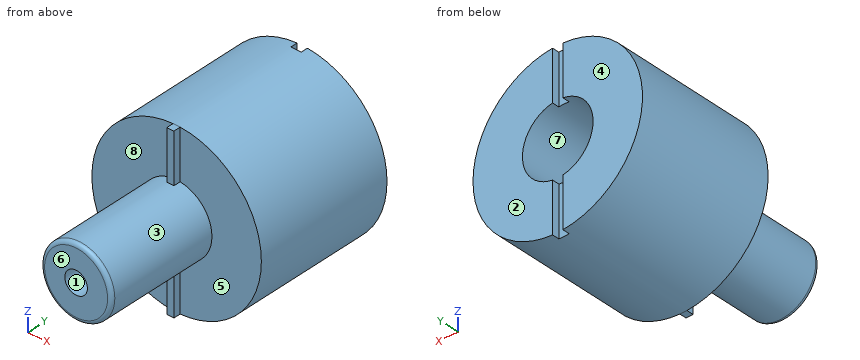
from build123d import *

# Parameters (mm, degrees)
F0_R      = 19.05
F1_DEPTH  = 31.75
F2_R      = 7.9375
F3_DEPTH  = 25.4
F4_R      = 0.8584943428
F6_DEPTH  = 1.5875
F8_DEPTH  = 1.5875
F11_R     = 7.9375
F12_DEPTH = 25.4
F9_R      = 2.54
F13_DEPTH = 31.75
F14_DEPTH = 1.5875


with BuildPart() as f1:
    # F0 (on Front) → F1 (new body)
    with BuildSketch(Plane.XZ):
        Circle(F0_R)
    extrude(amount=F1_DEPTH)

    # F2 (on face) → F3 (join)
    with BuildSketch(Plane.XZ.offset(31.75)):
        Circle(F2_R)
    extrude(amount=F3_DEPTH)

    # F4
    f4_edges = [f1.edges().sort_by_distance(p)[0] for p in [
        (-7.9375, -57.15, 0),
    ]]
    fillet(f4_edges, radius=F4_R)

    # F5 (on face) → F6 (join)
    with BuildSketch(Plane.XZ.offset(31.75)):
        with BuildLine():
            Line((0.79375, 19.0334563581), (-0.79375, 19.0334563581))
            Line((-0.79375, 19.0334563581), (-0.79375, 7.897712782))
            ThreePointArc((-0.79375, 7.897712782), (0, 7.9375), (0.79375, 7.897712782))
            Line((0.79375, 7.897712782), (0.79375, 19.0334563581))
        make_face()
    extrude(amount=F6_DEPTH)

    # F7 (on face) → F8 (join)
    with BuildSketch(Plane.XZ.offset(31.75)):
        with BuildLine():
            Line((-0.79375, -7.897712782), (-0.79375, -19.0334563581))
            Line((-0.79375, -19.0334563581), (0.79375, -19.0334563581))
            Line((0.79375, -19.0334563581), (0.79375, -7.897712782))
            ThreePointArc((0.79375, -7.897712782), (0, -7.9375), (-0.79375, -7.897712782))
        make_face()
    extrude(amount=F8_DEPTH)

    # F11 (on face) → F12 (cut)
    with BuildSketch(Plane(origin=(0, 0, 0), x_dir=(-1, 0, 0), z_dir=(0, 1, 0))):
        Circle(F11_R)
    extrude(amount=-F12_DEPTH, mode=Mode.SUBTRACT)

    # F9 (on face) → F13 (cut)
    with BuildSketch(Plane.XZ.offset(57.15)):
        Circle(F9_R)
    extrude(amount=-F13_DEPTH, mode=Mode.SUBTRACT)

    # F10 (on face) → F14 (cut)
    with BuildSketch(Plane(origin=(0, 0, 0), x_dir=(-1, 0, 0), z_dir=(0, 1, 0))):
        with BuildLine():
            ThreePointArc((1.1575095176, 19.0148013851), (0, 19.05), (-1.1575095176, 19.0148013851))
            Line((-1.1575095176, 19.0148013851), (-1.1575095176, -19.0148013851))
            ThreePointArc((-1.1575095176, -19.0148013851), (0, -19.05), (1.1575095176, -19.0148013851))
            Line((1.1575095176, -19.0148013851), (1.1575095176, 19.0148013851))
        make_face()
    extrude(amount=-F14_DEPTH, mode=Mode.SUBTRACT)


solid = f1.part
The model under review builds one solid part; all positions refer to its coordinate system, in mm. Face numbers are marked on the shaded views. A direction names the side the tool comes from. Give positions to 0.01 mm unless a question says otherwise; leave off trailing zeros. Loops run counter-clockwise (first coordinate to the right, second up) from the corner with the lowest first, then second, coordinate; pieces in that order, holes last. Notation, with made-up numbers: (-25, -3.75) -> (31, -3.75) arc R19 ccw to (31, 9.25) -> close; hole circle Ø5 at (44, 2.5). An arc over 180 degrees is marked (long way). Put each result on its own line as item: value. Start each with the question number.
1. Mouldability with a two-part tool opening along Z and no side actions: class the marked faces 1, 2 and 3 as released by +Z, released by -Z, zero draft, split by the parting line, or undercut.
2. We need section B-B on z = 0. State the section outline as (x, y) points.
3. Clearance check with flat-ended pins moving along their axes: P1, Ø9.5, axis at x = 0, z = 0, coming from the +Y side; P2, Ø9, axis at x = -14, z = 8.5, coming from the -Y side; P3, Ø0.7, axis at x = -0.5, z = 15, coming from the +Y side. State where each tip first meets the part, or that it passes through.
4. Wall thickness on probe 1 along Z at (x, y) = (0, -49); probe 2 along Z at (x, y) = (0, -8): over which ranges is each line inside the solid? List them lowest first.
5. For the marked faces 4, 5, 6, 7 and 8, list the 3-axis set-ups (+Z, -Z, +X, -X, +Y, -Y) from which the entire face can be reached by the end or side of a thin tool; tool diameter is ignored.
6. We need section D-D on z = -9. State the section outline as (x, y) points, then the cut area to 3 significant figures.
Determined:
1. face 1: undercut
1. face 2: zero draft
1. face 3: split by the parting line
2. outline: (-19.05, -31.75) -> (-7.94, -31.75) -> (-7.94, -56.29) arc R0.86 ccw to (-7.08, -57.15) -> (-2.54, -57.15) -> (-2.54, -25.4) -> (-7.94, -25.4) -> (-7.94, 0) -> (-19.05, 0) -> close; (2.54, -57.15) -> (7.08, -57.15) arc R0.86 ccw to (7.94, -56.29) -> (7.94, -31.75) -> (19.05, -31.75) -> (19.05, 0) -> (7.94, 0) -> (7.94, -25.4) -> (2.54, -25.4) -> close
3. P1: y = -25.4
3. P2: y = -31.75
3. P3: y = -1.59
4. probe 1: -7.94 to -2.54, 2.54 to 7.94
4. probe 2: -19.05 to -7.94, 7.94 to 19.05
5. face 4: +Z, -Z, +X, -X, +Y
5. face 5: +X, -Y
5. face 6: +Z, -Z, +X, -X, -Y
5. face 7: +Y
5. face 8: -X, -Y
6. outline: (-16.79, -31.75) -> (-0.79, -31.75) -> (-0.79, -33.34) -> (0.79, -33.34) -> (0.79, -31.75) -> (16.79, -31.75) -> (16.79, 0) -> (1.16, 0) -> (1.16, -1.59) -> (-1.16, -1.59) -> (-1.16, 0) -> (-16.79, 0) -> close
6. area: 1,070 mm^2
